Verification items for the finished model (mm, model axes). A direction names the side the tool comes from. Coordinates: 2 decimals unless noted, no trailing zeros. Write each loop counter-clockwise with the first axis right and the second up, starting at its lowest first coordinate (ties: lowest second). Pieces come first, ordered by that corner, then holes. Notation, with made-up numbers: (8.25, 86.25) -> (40.25, 86.25) arc R21 ccw to (40.25, 118.25) -> close; hole circle Ø1 at (-24.75, -0.5). An arc over 180 degrees is marked (long way). Answer in a Markdown table with one row per item.
```python
from build123d import *

# Parameters (mm, degrees)
SKETCH1_R           = 13
BOSS_EXTRUDE1_DEPTH = 1
SKETCH16_R          = 13
BOSS_EXTRUDE3_DEPTH = 1
SKETCH19_R          = 1
BOSS_EXTRUDE4_DEPTH = 29.8
SKETCH18_W          = 22
SKETCH18_H          = 22
CUT_EXTRUDE6_DEPTH  = 3.7
SKETCH21_R          = 11
CUT_EXTRUDE7_DEPTH  = 3.7
SKETCH22_R          = 11
CUT_EXTRUDE8_DEPTH  = 3.7
SKETCH23_R          = 11
CUT_EXTRUDE9_DEPTH  = 3.7
SKETCH24_R          = 19.921792127
CUT_EXTRUDE10_DEPTH = 1
SKETCH25_R          = 36.182885583
CUT_EXTRUDE11_DEPTH = 1
BOSS_EXTRUDE5_START = 2
BOSS_EXTRUDE5_DEPTH = 2
SKETCH27_R          = 1
BOSS_EXTRUDE6_DEPTH = 2
SKETCH28_R          = 15.857434306
CUT_EXTRUDE12_DEPTH = 26.1


with BuildPart() as part:
    # Sketch1 → Boss-Extrude1 (new body)
    with BuildSketch(Plane(origin=(0, 0, 0), x_dir=(1, 0, 0), z_dir=(0, 1, 0))):
        with Locations(Location((0, 0, 0), (0, 0, 270))):
            Circle(SKETCH1_R)
    extrude(amount=BOSS_EXTRUDE1_DEPTH)



with BuildPart() as body_2:
    # Sketch16 → Boss-Extrude3 (new body)
    with BuildSketch(Plane(origin=(0, 30.8, 0), x_dir=(1, 0, 0), z_dir=(0, 1, 0))):
        with Locations(Location((0, 0, 0), (0, 0, 270))):
            Circle(SKETCH16_R)
    extrude(amount=BOSS_EXTRUDE3_DEPTH)


with BuildPart() as part_1:
    add(part.part)

    add(body_2.part)  # Boss-Extrude4 merges body 2
    # Sketch19 → Boss-Extrude4 (add)
    with BuildSketch(Plane(origin=(0, 1, 0), x_dir=(1, 0, 0), z_dir=(0, 1, 0))):
        with Locations(Location((0, 11, 0), (0, 0, 270))):
            Circle(SKETCH19_R)
    extrude(amount=BOSS_EXTRUDE4_DEPTH)

    # Sketch18 → Cut-Extrude6 (cut)
    with BuildSketch(Plane(origin=(0, 4.7, 0), x_dir=(1, 0, 0), z_dir=(0, 1, 0))):
        Rectangle(SKETCH18_W, SKETCH18_H)
    extrude(amount=-CUT_EXTRUDE6_DEPTH, mode=Mode.SUBTRACT)

    # Sketch21 → Cut-Extrude7 (cut)
    with BuildSketch(Plane(origin=(0, 13.4, 0), x_dir=(1, 0, 0), z_dir=(0, 1, 0))):
        Circle(SKETCH21_R)
    extrude(amount=-CUT_EXTRUDE7_DEPTH, mode=Mode.SUBTRACT)

    # Sketch22 → Cut-Extrude8 (cut)
    with BuildSketch(Plane(origin=(0, 22.1, 0), x_dir=(1, 0, 0), z_dir=(0, 1, 0))):
        Circle(SKETCH22_R)
    extrude(amount=-CUT_EXTRUDE8_DEPTH, mode=Mode.SUBTRACT)

    # Sketch23 → Cut-Extrude9 (cut)
    with BuildSketch(Plane(origin=(0, 30.8, 0), x_dir=(1, 0, 0), z_dir=(0, 1, 0))):
        Circle(SKETCH23_R)
    extrude(amount=-CUT_EXTRUDE9_DEPTH, mode=Mode.SUBTRACT)

    # Sketch24 → Cut-Extrude10 (cut)
    with BuildSketch(Plane(origin=(0, 31.8, 0), x_dir=(1, 0, 0), z_dir=(0, 1, 0))):
        Circle(SKETCH24_R)
    extrude(amount=-CUT_EXTRUDE10_DEPTH, mode=Mode.SUBTRACT)

    # Sketch25 → Cut-Extrude11 (cut)
    with BuildSketch(Plane(origin=(0, 1, 0), x_dir=(1, 0, 0), z_dir=(0, 1, 0))):
        Circle(SKETCH25_R)
    extrude(amount=-CUT_EXTRUDE11_DEPTH, mode=Mode.SUBTRACT)

    # Sketch26 → Boss-Extrude5 (add)
    with BuildSketch(Plane(origin=(0, 30.8, 0), x_dir=(1, 0, 0), z_dir=(0, 1, 0)).offset(BOSS_EXTRUDE5_START)):
        with BuildLine():
            ThreePointArc((-0.998966408, 10.954545455), (0, 11), (0.998966408, 10.954545455))
            ThreePointArc((0.998966408, 10.954545455), (0, 12), (-0.998966408, 10.954545455))
        make_face()
        with BuildLine():
            ThreePointArc((0.998966408, 10.954545455), (0.999741569, 10.977266852), (1, 11))
            ThreePointArc((1, 11), (-0.022733148, 11.999741569), (-0.998966408, 10.954545455))
            ThreePointArc((-0.998966408, 10.954545455), (0, 11), (0.998966408, 10.954545455))
        make_face()
        with BuildLine():
            ThreePointArc((0.998966408, 10.954545455), (0, 11), (-0.998966408, 10.954545455))
            ThreePointArc((-0.998966408, 10.954545455), (0, 10), (0.998966408, 10.954545455))
        make_face()
    extrude(amount=-BOSS_EXTRUDE5_DEPTH)

    # Sketch27 → Boss-Extrude6 (add)
    with BuildSketch(Plane.XZ.offset(-1)):
        with Locations(Location((0, -11, 0), (0, 0, 270))):
            Circle(SKETCH27_R)
    extrude(amount=BOSS_EXTRUDE6_DEPTH)

    # Sketch28 → Cut-Extrude12 (cut)
    with BuildSketch(Plane(origin=(0, 32.8, 0), x_dir=(1, 0, 0), z_dir=(0, 1, 0))):
        with Locations((-0.375221001, 0)):
            Circle(SKETCH28_R)
    extrude(amount=-CUT_EXTRUDE12_DEPTH, mode=Mode.SUBTRACT)


solid = part_1.part
```
1. Tool access check on faces 1 (the flat face through (0, 4.7, -10.6)), 2 (the cylindrical face through (-0.6, 2.9, -11.8)). Record the directions out of +Z, -Z, +X, -X, +Y, -Y that give a thin tool (end or side, any length) a straight path to the whole face; none if there is none.
Geometry says:
| item | result |
|---|---|
| face 1 | +Z, +X, -X |
| face 2 | +Y, -Y |
2. Mould release check, pull along Y, two halves, no side actions. Record for faces 3 (the flat face through (0, 6.7, -11)), 4 (the flat face through (0, -1, -11)), 5 (the flat face through (0, 1, -10.6)): released by +Y, released by -Y, zero draft, split by the parting line, or undercut.
Geometry says:
| item | result |
|---|---|
| face 3 | released by +Y |
| face 4 | released by -Y |
| face 5 | undercut |
3. Section check A-A, the plane z = -10.4. Record the boundary of the cut face in (x, y), plus the area to 3 significant figures.
Geometry says:
| item | result |
|---|---|
| outline | (-0.8, -1) -> (0.8, -1) -> (0.8, 1) -> (-0.8, 1) -> close; (-0.8, 4.7) -> (0.8, 4.7) -> (0.8, 6.7) -> (-0.8, 6.7) -> close |
| area | 6.40 mm^2 |
4. Thickness scan on line 1 (Y direction, x = -0.3, z = -10.55); line 2 (Z direction, x = -0.65, y = 6); line 3 (X direction, y = 3, z = -11.5). Record the ranges inside material, lowest first. Write a range as from..to.
Geometry says:
| item | result |
|---|---|
| line 1 | -1..1, 4.7..6.7 |
| line 2 | -11.76..-10.24 |
| line 3 | -0.87..0.87 |
5. Section check B-B, the plane x = 0.3. Record the boundary of the cut face in (y, z).
Geometry says:
| item | result |
|---|---|
| outline | (-1, -11.95) -> (6.7, -11.95) -> (6.7, -10.05) -> (4.7, -10.05) -> (4.7, -11) -> (1, -11) -> (1, -10.05) -> (-1, -10.05) -> close |
6. Section check D-D, the plane z = -10.85. Record the boundary of the cut face in (x, y), plus the area to 3 significant figures.
Geometry says:
| item | result |
|---|---|
| outline | (-0.99, -1) -> (0.99, -1) -> (0.99, 1) -> (-0.99, 1) -> close; (-0.99, 4.7) -> (0.99, 4.7) -> (0.99, 6.7) -> (-0.99, 6.7) -> close |
| area | 7.91 mm^2 |
7. Section check C-C, the plane y = 5.5. Record the boundary of the cut face in (x, z).
Geometry says:
| item | result |
|---|---|
| outline | circle Ø2 at (0, -11) |
